Geometry check sheet. Reference: the model listing, model coordinates, mm. A direction names the side the tool comes from. Coordinates: 2 decimals unless noted, no trailing zeros. Loops run counter-clockwise (first coordinate to the right, second up) from the corner with the lowest first, then second, coordinate; pieces in that order, holes last. Notation, with made-up numbers: (51.5, -6) - (83.5, -6) arc R22 cw to (83.5, 33) - close; hole circle Ø4 at (56.5, -34). An arc over 180 degrees is marked (long way). One line per item, written item: value.
from build123d import *

# Parameters (mm, degrees)
SKETCH1_W                  = 609.6
SKETCH1_H                  = 1219.2
BOSS_EXTRUDE1_DEPTH        = 5.5
BOSS_EXTRUDE2_DEPTH        = 6.35
F_5_3_5_3_DIAMETER_HOLE1_D = 5.3
CUT_EXTRUDE1_REACH         = 1365.159
CUT_EXTRUDE2_DEPTH         = 994.074837311
BOSS_EXTRUDE3_DEPTH        = 10


with BuildPart() as part:
    # Sketch1 → Boss-Extrude1 (new body)
    with BuildSketch(Plane(origin=(0, 0, 0), x_dir=(1, 0, 0), z_dir=(0, 1, 0))):
        with Locations((304.8, 609.6)):
            Rectangle(SKETCH1_W, SKETCH1_H)
    extrude(amount=BOSS_EXTRUDE1_DEPTH)

    # Sketch3 → Boss-Extrude2 (add)
    with BuildSketch(Plane(origin=(0, 5.5, 0), x_dir=(1, 0, 0), z_dir=(0, 1, 0))):
        Polygon((387.35, 0), (387.35, 914.4), (0, 914.4), (0, 1219.2), (609.6, 1219.2), (609.6, 0), align=None)
    extrude(amount=BOSS_EXTRUDE2_DEPTH)

    # 5.3 _5.3_ Diameter Hole1 (through all)
    with Locations(Plane(origin=(0, 5.5, 0), x_dir=(1, 0, 0), z_dir=(0, 1, 0))):
        with Locations((19.05, 895.35), (44.45, 895.35), (69.85, 895.35), (19.05, 869.95), (19.05, 844.55), (19.05, 457.2), (19.05, 69.85), (19.05, 44.45), (19.05, 19.05), (44.45, 19.05), (69.85, 19.05), (190.5, 19.05), (311.15, 19.05), (336.55, 19.05), (361.95, 19.05), (361.95, 44.45), (361.95, 69.85), (361.95, 457.2), (361.95, 844.55), (361.95, 869.95), (361.95, 895.35), (336.55, 895.35), (311.15, 895.35), (190.5, 895.35)):
            Hole(F_5_3_5_3_DIAMETER_HOLE1_D / 2)

    # Sketch7 → Cut-Extrude1 (cut, up to next)
    with BuildSketch(Plane(origin=(0, 11.85, 0), x_dir=(1, 0, 0), z_dir=(0, 1, 0)), mode=Mode.PRIVATE) as cut_extrude1_sk1:
        Polygon((0, 1219.2), (0, 914.4), (387.35, 914.4), (387.35, 0), (609.6, 0), (609.6, 1219.2), align=None)
    cut_extrude1_tool1 = extrude(cut_extrude1_sk1.sketch, amount=-CUT_EXTRUDE1_REACH, mode=Mode.PRIVATE) & part.part
    add(cut_extrude1_tool1.solids().sort_by_distance((405.973507, 11.85, -748.352239))[0], mode=Mode.SUBTRACT)

    # Sketch8 → Cut-Extrude2 (cut, through all)
    with BuildSketch(Plane(origin=(0, 5.5, 0), x_dir=(1, 0, 0), z_dir=(0, 1, 0))):
        with BuildLine():
            ThreePointArc((189.987652462, 16.45), (187.85, 19.05), (189.987652462, 21.65))
            Line((189.987652462, 21.65), (165.1, 21.65))
            ThreePointArc((165.1, 21.65), (162.5, 19.05), (165.1, 16.45))
            Line((165.1, 16.45), (189.987652462, 16.45))
        make_face()
        with BuildLine():
            ThreePointArc((190.5, 21.65), (187.9, 19.05), (190.5, 16.45))
            ThreePointArc((190.5, 16.45), (193.1, 19.05), (190.5, 21.65))
        make_face()
        with BuildLine():
            Line((215.9, 21.65), (191.012347538, 21.65))
            ThreePointArc((191.012347538, 21.65), (192.546975937, 20.732970443), (193.15, 19.05))
            ThreePointArc((193.15, 19.05), (192.546975937, 17.367029557), (191.012347538, 16.45))
            Line((191.012347538, 16.45), (215.9, 16.45))
            ThreePointArc((215.9, 16.45), (218.5, 19.05), (215.9, 21.65))
        make_face()
        with BuildLine():
            ThreePointArc((165.1, 897.95), (162.5, 895.35), (165.1, 892.75))
            Line((165.1, 892.75), (189.987652462, 892.75))
            ThreePointArc((189.987652462, 892.75), (187.85, 895.35), (189.987652462, 897.95))
            Line((189.987652462, 897.95), (165.1, 897.95))
        make_face()
        with BuildLine():
            ThreePointArc((190.5, 892.75), (187.9, 895.35), (190.5, 897.95))
            ThreePointArc((190.5, 897.95), (193.1, 895.35), (190.5, 892.75))
        make_face()
        with BuildLine():
            ThreePointArc((193.15, 895.35), (192.546975937, 893.667029557), (191.012347538, 892.75))
            Line((191.012347538, 892.75), (215.9, 892.75))
            ThreePointArc((215.9, 892.75), (218.5, 895.35), (215.9, 897.95))
            Line((215.9, 897.95), (191.012347538, 897.95))
            ThreePointArc((191.012347538, 897.95), (192.546975937, 897.032970443), (193.15, 895.35))
        make_face()
    extrude(amount=-CUT_EXTRUDE2_DEPTH, mode=Mode.SUBTRACT)

    # Sketch9 → Boss-Extrude3 (add)
    with BuildSketch(Plane.XZ):
        Polygon((0, -1219.2), (609.6, -1219.2), (609.6, 0), (387.35, 0), (387.35, -914.4), (0, -914.4), align=None)
    extrude(amount=-BOSS_EXTRUDE3_DEPTH)


solid = part.part
(1) Cross-section at B-B on z = -728. Record the cut outline in (x, y).
Reply:
outline: (0, 0) - (609.6, 0) - (609.6, 10) - (387.35, 10) - (387.35, 5.5) - (0, 5.5) - close
(2) Material ranges on probe 1 along X at (y, z) = (3.8, -844.55); probe 2 along Z at (x, y) = (336.55, 1.6); probe 3 along Z at (x, y) = (344, 8), recorded low to high. Write a range as from..to.
Reply:
probe 1: 0..16.4, 21.7..359.3, 364.6..609.6
probe 2: -1219.2..-898, -892.7..-21.7, -16.4..0
probe 3: -1219.2..-914.4
(3) Access from +Z, -Z, +X, -X, +Y, -Y to the whole of each face (thin tool, end or side, straight path). Record for faces 1 (the face through (191, 5.5, -464)), 2 (the face through (301, 0, -601)).
Reply:
face 1: +Z, -X, +Y
face 2: +Z, -Z, +X, -X, -Y
(4) Go/stop test with a flat-tipped pin: pin 1 Ø6 at (x, z) = (311.15, -19.05) entering from +Y. Record where the tip stops, or that it passes through.
Reply:
pin 1: y = 5.5
(5) Cross-section at A-A on y = 7.75. Record the cut outline in (x, z).
Reply:
outline: (0, -1219.2) - (609.6, -1219.2) - (609.6, 0) - (387.35, 0) - (387.35, -914.4) - (0, -914.4) - close
